Check sheet for the modelled part. Datum: model origin and axes. Units: mm. Face numbers are marked on the shaded views. A direction names the side the tool comes from. Round coordinates to 2 decimals unless told otherwise and drop trailing zeros. Loops run counter-clockwise (first coordinate to the right, second up) from the corner with the lowest first, then second, coordinate; pieces in that order, holes last. Notation, with made-up numbers: (51.5, -24.5) -> (74.5, -24.5) arc R19 ccw to (74.5, -20.5) -> close; hole circle Ø9 at (74, 0.5). An arc over 180 degrees is marked (long way). Use one line per item in the form item = value. Start each with the question number.
(1) Material ranges on probe 1 along X at (y, z) = (0, -3.55); probe 2 along Y at (x, z) = (0, -14.5), recorded low to high. Write a range as [from, to].
(2) Set-up check for the marked faces 1 and 2: record each of +Z, -Z, +X, -X, +Y, -Y from which the full face is reachable in a straight line by a thin tool's end or side.
(3) Go/stop test with flat-tipped pins: pin 1 (9 mm diameter, centred on x = -1, y = 1, fed in from +Z) (1 decimal); pin 2 (1 mm diameter, centred on y = -7.5, z = -16, fed in from -X); pin 3 (2 mm diameter, centred on y = 2.5, z = -15, fed in from +X); pin 4 (5 mm diameter, centred on x = -12.5, z = -6, fed in from +Y). Record where each tip stops, or that it passes through.
(4) Sectioned sample at D-D (z = -17.75). Record the cut outline in (x, y).
(5) Sectioned sample at C-C (y = 8). Record the cut outline in (x, z), and give its area (3 significant figures).
(6) Draft check along X on the marked faces 3, 4, 5 and 6. Enter one of: released by +X, released by -X, zero draft, split by the parting line, or undercut.
(7) Sectioned sample at A-A (y = 0). Record the cut outline in (x, z), and give its area (3 significant figures).
(8) Sectioned sample at B-B (x = 5). Record the cut outline in (y, z).
from build123d import *

# Parameters (mm, degrees)
HOLE_WIZARD_M16_1_D = 14


with BuildPart() as part:
    # 草圖1 → 旋轉1 (revolve)
    with BuildSketch(Plane(origin=(0, 0, 0), x_dir=(0, 0, -1), z_dir=(1, 0, 0))):
        Polygon((5, 0), (5, 9), (0, 9), (0, 16), (24, 16), (24, 0), align=None)
    revolve(axis=Axis((0, 0, -24), (0, 0, 1)))

    # 草圖2 → 除料-旋轉1 (revolve, cut)
    with BuildSketch(Plane(origin=(0, 0, 0), x_dir=(0, 0, -1), z_dir=(1, 0, 0))):
        Polygon((3.7183072, 19.324474935), (10, 19.324474935), (10, 13.5), (3.7183072, 17.126737029), align=None)
    revolve(axis=Axis((0, 11.187716982, -10), (0, 1, 0)), mode=Mode.SUBTRACT)

    # M16 螺紋孔1 (through all)
    with Locations(Plane.XY.offset(-5)):
        with Locations((0, 0)):
            Hole(HOLE_WIZARD_M16_1_D / 2)


solid = part.part
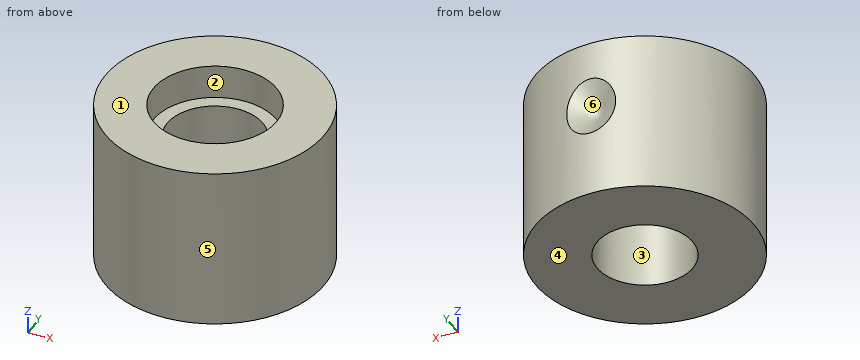
Checks:
q1.probe_1 = [-16, -9], [9, 16]
q1.probe_2 = [-16, -7], [7, 16]
q2.face_1 = +Z, +X, -X, +Y, -Y
q2.face_2 = +Z
q3.pin_1 = through
q3.pin_2 = -14.39
q3.pin_3 = 15.93
q3.pin_4 = 12.49
q4.outline = circle Ø32 at (0, 0); hole circle Ø14 at (0, 0)
q5.outline = (-13.86, -24) -> (13.86, -24) -> (13.86, 0) -> (4.12, 0) -> (4.12, -5) -> (-4.12, -5) -> (-4.12, 0) -> (-13.86, 0) -> close
q5.area = 624 mm2
q6.face_3 = undercut
q6.face_4 = zero draft
q6.face_5 = split by the parting line
q6.face_6 = undercut
q7.outline = (-16, -24) -> (-7, -24) -> (-7, -5) -> (-9, -5) -> (-9, 0) -> (-16, 0) -> close; (7, -24) -> (16, -24) -> (16, 0) -> (9, 0) -> (9, -5) -> (7, -5) -> close
q7.area = 412 mm2
q8.outline = (-15.2, -24) -> (-4.9, -24) -> (-4.9, -5) -> (-7.48, -5) -> (-7.48, 0) -> (-15.2, 0) -> close; (4.9, -24) -> (15.2, -24) -> (15.2, 0) -> (7.48, 0) -> (7.48, -5) -> (4.9, -5) -> close
